Autodesk Inventor part; units mm, degrees
ref_plane "YZ Plane" through (0, 0, 0) normal (1, 0, 0) x (0, 1, 0)
ref_plane "XZ Plane" through (0, 0, 0) normal (0, 1, 0) x (-1, 0, 0)
ref_plane "XY Plane" through (0, 0, 0) normal (0, 0, 1) x (1, 0, 0)
sketch "Sketch1" plane through (0, 0, 0) normal (0, 1, 0) x (-1, 0, 0)
  line L0 (0, 0) -> (0, -314.325)
  line L1 (0, -314.325) -> (192.0875, -314.325)
  line L2 (192.0875, -314.325) -> (192.0875, -506.4125)
  line L3 (192.0875, -506.4125) -> (506.4125, -506.4125)
  line L4 (506.4125, -506.4125) -> (506.4125, -314.325)
  line L5 (506.4125, -314.325) -> (698.5, -314.325)
  line L6 (698.5, -314.325) -> (698.5, 0)
  line L7 (698.5, 0) -> (506.4125, 0)
  line L8 (506.4125, 0) -> (506.4125, 192.0875)
  line L9 (506.4125, 192.0875) -> (192.0875, 192.0875)
  line L10 (192.0875, 192.0875) -> (192.0875, 0)
  line L11 (192.0875, 0) -> (0, 0)
  line L12 (698.5, 192.0875) -> (0, 192.0875) construction
  line L13 (0, 192.0875) -> (0, -506.4125) construction
  line L14 (0, -506.4125) -> (698.5, -506.4125) construction
  line L15 (698.5, -506.4125) -> (698.5, 192.0875) construction
  dimension "d0" = 698.5
  dimension "d1" = 192.0875
extrude "Plate1" add sketch "Sketch1" along normal blind 3.175
sketch "Sketch2" plane through (0, 3.175, 0) normal (0, 1, 0) x (1, 0, 0)
  line L0 (-506.4125, 506.4125) -> (-192.0875, 506.4125)
  line L1 (0, 314.325) -> (0, 0)
  line L2 (-192.0875, -192.0875) -> (-506.4125, -192.0875)
  line L3 (-698.5, 0) -> (-698.5, 314.325)
  line L4 (-506.4125, 314.325) -> (-506.4125, 506.4125)
  line L5 (-192.0875, 506.4125) -> (-192.0875, 314.325)
  line L6 (-698.5, 314.325) -> (-506.4125, 314.325)
  line L7 (-506.4125, 0) -> (-698.5, 0)
  line L8 (-349.25, 506.4125) -> (-349.25, -192.0875) construction
  line L9 (-698.5, 157.1625) -> (0, 157.1625) construction
  point P0 (-481.0125, 493.7125)
  point P1 (-430.2125, 493.7125)
  point P2 (-268.2875, 493.7125)
  point P3 (-217.4875, 493.7125)
  point P4 (-12.7, 288.925)
  point P5 (-12.7, 238.125)
  point P6 (-12.7, 76.2)
  point P7 (-12.7, 25.4)
  point P8 (-217.4875, -179.3875)
  point P9 (-268.2875, -179.3875)
  point P10 (-430.2125, -179.3875)
  point P11 (-481.0125, -179.3875)
  point P12 (-685.8, 25.4)
  point P13 (-685.8, 76.2)
  point P14 (-685.8, 238.125)
  point P15 (-685.8, 288.925)
  point P16 (-349.25, 493.7125)
  point P17 (-349.25, -179.3875)
  point P18 (-685.8, 157.1625)
  point P19 (-12.7, 157.1625)
  dimension "d3" = 12.7
  dimension "d4" = 12.7
  dimension "d5" = 12.7
  dimension "d6" = 12.7
  dimension "d7" = 25.4
  dimension "d8" = 50.8
  dimension "d9" = 25.4
  dimension "d10" = 50.8
  dimension "d11" = 25.4
  dimension "d12" = 50.8
  dimension "d13" = 25.4
  dimension "d14" = 50.8
hole "Hole1" at (-685.8, 3.175, -288.925) at (-685.8, 3.175, -238.125) at (-685.8, 3.175, -76.2) at (-685.8, 3.175, -25.4) at (-481.0125, 3.175, 179.3875) at (-430.2125, 3.175, 179.3875) at (-268.2875, 3.175, 179.3875) at (-217.4875, 3.175, 179.3875) at (-12.7, 3.175, -25.4) at (-12.7, 3.175, -76.2) at (-12.7, 3.175, -238.125) at (-12.7, 3.175, -288.925) at (-217.4875, 3.175, -493.7125) at (-268.2875, 3.175, -493.7125) at (-430.2125, 3.175, -493.7125) at (-481.0125, 3.175, -493.7125) at (-685.8, 3.175, -157.1625) at (-349.25, 3.175, 179.3875) at (-12.7, 3.175, -157.1625) at (-349.25, 3.175, -493.7125) direction (0, -1, 0) diameter 4.0894 end through all
sketch "Sketch3" plane through (0, 3.175, 0) normal (0, 1, 0) x (1, 0, 0)
  circle A0 centre (-12.7, 25.4) radius 2.0447 construction
sketch "Sketch4" plane through (0, 3.175, 0) normal (0, 1, 0) x (1, 0, 0)
  circle A0 centre (-12.7, 76.2) radius 2.0447 construction
sketch "Sketch5" plane through (0, 3.175, 0) normal (0, 1, 0) x (1, 0, 0)
  circle A0 centre (-456.9079, 207.9586) radius 2.5
  circle A1 centre (-241.0079, 207.9586) radius 2.5
  circle A2 centre (-241.0079, 106.3586) radius 2.5
  circle A3 centre (-456.9079, 106.3586) radius 2.5
  point P0 (0, 0)
hole "Hole2" at (-456.9079, 3.175, -207.9586) at (-241.0079, 3.175, -207.9586) at (-456.9079, 3.175, -106.3586) at (-241.0079, 3.175, -106.3586) direction (0, -1, 0) diameter 5.1054 end through all
sketch "Sketch6" plane through (0, 3.175, 0) normal (0, 1, 0) x (1, 0, 0)
  circle A0 centre (-475.0703, -29.3212) radius 2.5
  circle A1 centre (-436.9703, -29.3212) radius 2.5
  circle A2 centre (-475.0703, -130.9212) radius 2.5
  circle A3 centre (-436.9703, -130.9212) radius 2.5
  point P0 (0, 0)
hole "Hole3" at (-475.0703, 3.175, 130.9212) at (-436.9703, 3.175, 130.9212) at (-475.0703, 3.175, 29.3212) at (-436.9703, 3.175, 29.3212) direction (0, -1, 0) diameter 5.1054 end through all
sketch "Sketch8" plane through (0, 3.175, 0) normal (0, 1, 0) x (1, 0, 0)
  circle A0 centre (-139.7, 262.7312) radius 2.0447
  circle A1 centre (-38.1, 262.7312) radius 2.0447
  circle A2 centre (-139.7, 51.5937) radius 2.0447
  circle A3 centre (-38.1, 51.5937) radius 2.0447
  circle A4 centre (-209.2008, 207.9625) radius 2.0447
  circle A5 centre (-209.2008, 106.3625) radius 2.0447
  point P0 (0, 0)
hole "Hole4" at (-139.7, 3.175, -262.7312) at (-38.1, 3.175, -262.7312) at (-139.7, 3.175, -51.5937) at (-38.1, 3.175, -51.5937) at (-209.2008, 3.175, -207.9625) at (-209.2008, 3.175, -106.3625) direction (0, -1, 0) diameter 4.0894 end through all
equation "\"d0\" = DrivebaseLength"
equation "\"d1\" = PlateCut"
equation "\"d20\" = Thickness"
equation "\"d27\" = Thickness"
equation "\"d41\" = Thickness"
equation "\"d2\" = Thickness"
equation "\"BendRadius\" = 1.5 * Thickness"
equation "\"BendReliefWidth\" = Thickness"
equation "\"BendReliefDepth\" = 0.5 * Thickness"
equation "\"CornerReliefSize\" = 4 * Thickness"
equation "\"MinimumRemnant\" = 2 * Thickness"
equation "\"TransitionRadius\" = BendRadius"
equation "\"JacobiRadiusSize\" = BendRadius"
equation "\"GapSize\" = Thickness"
equation "\"DrivebaseLength\" = 698.5"
equation "\"DrivebaseWidth\" = 698.5"
equation "\"LengthOfTube\" = 482.6"
equation "\"ModuleSize\" = 169.8625"
equation "\"EdgeModuleToHole\" = 61.9125"
equation "\"ModuleSpace\" = 107.95"
equation "\"HoleLength1\" = 6.35"
equation "\"HoleLength2\" = 31.75"
equation "\"HoleLength3\" = 57.15"
equation "\"HoleLength4\" = 425.45"
equation "\"HoleLength5\" = 450.85"
equation "\"HoleLength6\" = 476.25"
equation "\"HoleWidth\" = 12.7"
equation "\"ModuleLength\" = 190.5"
equation "\"PlateCut\" = 192.0875"
equation "\"Rivet1\" = 109.5375"
equation "\"Rivet2\" = 160.3375"
equation "\"Rivet4\" = 322.2625"
equation "\"Rivet3\" = 241.3"
equation "\"Rivet5\" = 373.0625"
properties part number "200510" material "Aluminum 5052 H32"
Can you work these out from the model? Positions are in its coordinate system, mm. Give positions to 0.01 mm unless a question says otherwise; leave off trailing zeros. Loops run counter-clockwise (first coordinate to the right, second up) from the corner with the lowest first, then second, coordinate; pieces in that order, holes last. Notation, with made-up numbers: (12.25, -10.5) -> (53.25, -10.5) arc R18 cw to (53.25, 4.5) -> close; hole circle Ø8 at (-29.75, -20). An arc over 180 degrees is marked (long way). Write item = value, one per line.
1) Will these pins go through, and if not, where does the flat tip stop? pin 1 (1 mm diameter, centred on y = 1, z = 67.5, fed in from +X); pin 2 (3.5 mm diameter, centred on x = -217.49, z = -493.71, fed in from +Y); pin 3 (1.6 mm diameter, centred on x = -61, y = 1.5, fed in from +Z).
Check result:
pin_1 = -192.09
pin_2 = through
pin_3 = 0
2) Suppose I cut it at C-C on z = -403. Write out the boundary of the cut face in (x, y) (1 decimal), then the cut area to 3 significant figures.
Check result:
outline = (-506.4, 0) -> (-192.1, 0) -> (-192.1, 3.2) -> (-506.4, 3.2) -> close
area = 998 mm2
3) Suppose I cut it at B-B on y = 2.65. Give the number of separate pieces and of enclosed holes in the cut face, then the cut area to 3 significant figures.
Check result:
separate_pieces = 1
enclosed_holes = 34
area = 340,000 mm2
4) Suppose I cut it at A-A on x = -546.5. Write out the boundary of the cut face in (y, z) (3 decimals), then the cut area to 3 significant figures.
Check result:
outline = (0, -314.325) -> (3.175, -314.325) -> (3.175, 0) -> (0, 0) -> close
area = 998 mm2
5) I need wall thicknesses on L1, parallel to Z at x = -350, y = 1.8; L2, parallel to Z at x = -38.1, y = 0.9 (1 decimal); L3, parallel to X at y = 2, z = -76.2. Which ranges of each line are inside material? Lowest first, please. Write a range as from..to.
Check result:
L1 = -506.41..-495.61, -491.81..177.49, 181.29..192.09
L2 = -314.3..-264.8, -260.7..-53.6, -49.5..0
L3 = -698.5..-687.84, -683.76..-14.74, -10.66..0
